Check sheet for the modelled part. Datum: model origin and axes. Units: mm. Round coordinates to 2 decimals unless told otherwise and drop trailing zeros. Order: outer loops, then holes, each group sorted by start corner. A loop starts at its lowest first (then second) coordinate and runs counter-clockwise, first axis right, second up. Notation, with made-up numbers: (44.5, 23) -> (49.5, 23) arc R15 cw to (49.5, 48) -> close; hole circle Ø8 at (10, -5). An arc over 180 degrees is marked (long way). Answer as CSV lines item,"result". Start each with the question number.
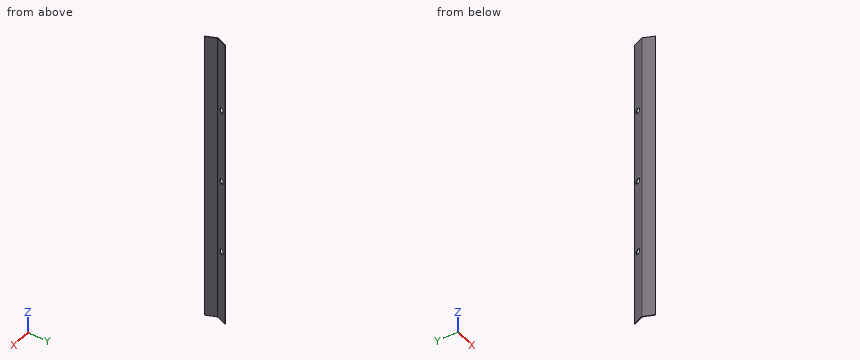
Autodesk Inventor part; units mm, degrees
ref_plane "YZ Plane" through (0, 0, 0) normal (1, 0, 0) x (0, 1, 0)
ref_plane "XZ Plane" through (0, 0, 0) normal (0, 1, 0) x (-1, 0, 0)
ref_plane "XY Plane" through (0, 0, 0) normal (0, 0, 1) x (1, 0, 0)
sketch "Sketch4" plane through (0, 0, 0) normal (0, 0, 1) x (1, 0, 0)
  line L0 (-202.056852, 202.056852) -> (0, 285.751541) construction
  line L1 (0, 285.751541) -> (202.056852, 202.056852) construction
  line L2 (202.056852, 202.056852) -> (285.751541, 0) construction
  line L3 (285.751541, 0) -> (202.056852, -202.056852) construction
  line L4 (202.056852, -202.056852) -> (0, -285.751541) construction
  line L5 (0, -285.751541) -> (-202.056852, -202.056852) construction
  line L6 (-202.056852, -202.056852) -> (-285.751541, 0) construction
  line L7 (-285.751541, 0) -> (-202.056852, 202.056852) construction
  line L8 (-285.11749, 1.530734) -> (-271.241389, 35.030606)
  line L9 (-285.11749, -1.530734) -> (-271.241389, -35.030606)
  arc A0 (-285.11749, 1.530734) -> (-285.11749, -1.530734) centre (-281.421972, 0) ccw
  point P0 (0, 0)
  point P1 (0, 0)
  point P2 (0, 0)
  dimension "d16" = 528
  dimension "d23" = 36.26
  dimension "d24" = 4
contour flange "Contour Flange1" sketch "Sketch4" thickness 2 bend radius 2 width 988.5 along (0, 0, -1) mid plane no both sides no wall seen from (-278.17944, 18.28067, 0) lies toward (0.9238795, -0.3826834, 0) curves L8 A0 L9
bend "Bend2"
corner "Corner2"
sketch "Sketch6" plane through (-285.11749, 1.530734, 0) normal (-0.9238795, 0.3826834, 0) x (0.3826834, 0.9238795, 0)
  circle A0 centre (19.22, 40.75) radius 5.5 construction
  circle A1 centre (19.22, 947.75) radius 5.5 construction
  line L0 (0, 0) -> (0, 988.5)
  line L1 (36.26, 988.5) -> (0, 988.5)
  line L2 (36.26, 0) -> (0, 0)
  line L3 (27.62, 942.900258) -> (19.22, 938.050515)
  line L4 (19.22, 938.050515) -> (10.82, 942.900258)
  line L5 (10.82, 942.900258) -> (10.82, 952.599742)
  line L6 (10.82, 952.599742) -> (19.22, 957.449485)
  line L7 (19.22, 957.449485) -> (27.62, 952.599742)
  line L8 (27.62, 952.599742) -> (27.62, 942.900258)
  line L9 (27.62, 35.900258) -> (19.22, 31.050515)
  line L10 (19.22, 31.050515) -> (10.82, 35.900258)
  line L11 (10.82, 35.900258) -> (10.82, 45.599742)
  line L12 (10.82, 45.599742) -> (19.22, 50.449485)
  line L13 (19.22, 50.449485) -> (27.62, 45.599742)
  line L14 (27.62, 45.599742) -> (27.62, 35.900258)
  point P0 (107.695526, 0)
  dimension "d36" = 11
  dimension "d41" = 11
  dimension "d93" = 19.22
  dimension "d94" = 40.75
  dimension "d95" = 19.22
  dimension "d96" = 40.75
  dimension "d98" = 16.8
  dimension "d99" = 16.8
extrude "Extrusion1" [suppressed]
sketch "Sketch13" plane through (-285.11749, 1.530734, 0) normal (-0.9238795, 0.3826834, 0) x (0.3826834, 0.9238795, 0)
  circle A0 centre (19.22, 494.25) radius 5.5 construction
  line L0 (36.26, 0) -> (36.26, 988.5)
  line L1 (36.26, 0) -> (0, 0)
  line L2 (27.62, 489.400258) -> (19.22, 484.550515)
  line L3 (19.22, 484.550515) -> (10.82, 489.400258)
  line L4 (10.82, 489.400258) -> (10.82, 499.099742)
  line L5 (10.82, 499.099742) -> (19.22, 503.949485)
  line L6 (19.22, 503.949485) -> (27.62, 499.099742)
  line L7 (27.62, 499.099742) -> (27.62, 489.400258)
  point P0 (107.695526, 0)
  point P1 (36.26, 494.25)
  point P2 (35, 910)
  point P3 (35, 1110)
  point P4 (18.13, 0)
  point P5 (27.62, 494.25)
  dimension "d83" = 11
  dimension "magic_d1" = 17.04
  dimension "d97" = 16.8
extrude "Extrusion7" cut sketch "Sketch13" against normal through all
pattern_linear "Rectangular Pattern5" count 3 spacing 250 along (0, 0, 1) of "Extrusion7" first direction both ways yes
equation "\"d16\" = Барабан_размер_по_плоскостям - Thickness"
equation "\"d24\" = BendRadius + Thickness"
equation "\"d41\" = d36"
equation "\"d95\" = d93"
equation "\"d96\" = d94"
equation "\"d99\" = d98"
equation "\"d25\" = Thickness"
equation "\"d26\" = BendReliefWidth"
equation "\"d27\" = BendReliefDepth"
equation "\"d28\" = MinimumRemnant"
equation "\"d29\" = TransitionRadius"
equation "\"d31\" = BendRadius"
equation "\"d33\" = CornerReliefSize"
equation "\"d34\" = GapSize"
equation "\"d35\" = JacobiRadiusSize"
equation "\"BendRadius\" = Thickness"
equation "\"BendReliefWidth\" = Thickness"
equation "\"BendReliefDepth\" = 0.5 * Thickness"
equation "\"CornerReliefSize\" = 4 * Thickness"
equation "\"MinimumRemnant\" = 2 * Thickness"
equation "\"TransitionRadius\" = BendRadius"
equation "\"JacobiRadiusSize\" = BendRadius"
equation "\"GapSize\" = Thickness"
properties part number "DMF 01 17 опора крышки v2.1_CPY" material "Stainless Steel AISI 304"
1) Material ranges on line 1 along Y through (x, z) = (-279.75, -514); line 2 along Y through (x, z) = (-281.75, -616); line 3 along X through (y, z) = (18.5, -530.5), recorded low to high.
2) Section check B-B on y = -10.5. Record the cut outline in (x, z), then the cut area to 3 significant figures.
3) Depth check by flat-ended pin: pin 1 Ø5 at (x, z) = (-275.5, -207) entering from -Y; pin 2 Ø4 at (x, z) = (-272.5, -777.5) entering from -Y; pin 3 Ø10 at (y, z) = (-20.5, -353) entering from +X. Enter the tip coordinate at first touch or a pass-through.
4) Section check A-A on z = -882.5. Record the cut outline in (x, y), then the cut area to 3 significant figures.
Solutions:
1,line 1,"y = -14.49 to -9.26, 9.26 to 14.49"
1,line 2,"y = -9.66 to -4.43, 4.43 to 9.66"
1,line 3,"x = -278.09 to -275.92"
2,outline,"(-281.4, -988.5) -> (-279.24, -988.5) -> (-279.24, 0) -> (-281.4, 0) -> close"
2,area,"2,140 mm^2"
3,pin 1,"stops at y = -30.78"
3,pin 2,"stops at y = -35.03"
3,pin 3,"stops at x = -273.02"
4,outline,"(-285.12, -1.53) -> (-271.24, -35.03) -> (-269.39, -34.27) -> (-283.27, -0.77) arc R2 cw to (-283.27, 0.77) -> (-269.39, 34.27) -> (-271.24, 35.03) -> (-285.12, 1.53) arc R4 ccw to start"
4,area,"150 mm^2"
